Geometry check sheet. Reference: drawing and pictorial views, mm from the part's lowest x, y, z. A direction names the side the tool comes from. Round coordinates to 2 decimals unless told otherwise and drop trailing zeros. Order: outer loops, then holes, each group sorted by start corner. A loop starts at its lowest first (then second) coordinate and runs counter-clockwise, first axis right, second up.
(1) Gauge pin test, flat ends, axial feed: P1, Ø12, axis at x = 15.5, y = 15.5, coming from the +Z side; P2, Ø1.5, axis at x = 29.5, z = 3, coming from the +Y side; P3, Ø4.5, axis at y = 7.5, z = 2.5, coming from the -X side; P4, Ø4, axis at x = 30, y = 5, coming from the -Z side. Record the tip position at first contact, or that the pin passes through.
(2) Cross-section at C-C on z = 5.5. Enter the section's corners in (x, y), and give its area (3 significant figures).
(3) Cross-section at B-B on x = 31.5. Enter the section's corners in (y, z).
(4) Cross-section at D-D on x = 9.5. Enter the section's corners in (y, z), and give its area (3 significant figures).
(5) Draft check along X on the marked faces 4, 5 and 6. Enter one of: pulls with the +X half, pulls with the -X half, needs draft (parallel to the pull), parting line crosses it, or undercut.
(6) Cross-section at A-A on z = 0.5. Enter the section's corners in (x, y).
(7) Thickness scan on L1, parallel to X at y = 9, z = 8; L2, parallel to Y at x = 30, z = 7.5; L3, parallel to X at y = 4, z = 1.75. Record the ranges inside material, lowest first.
(8) Set-up check for the marked faces 1, 2 and 3: record each of +Z, -Z, +X, -X, +Y, -Y from which the full face is reachable in a straight line by a thin tool's end or side.
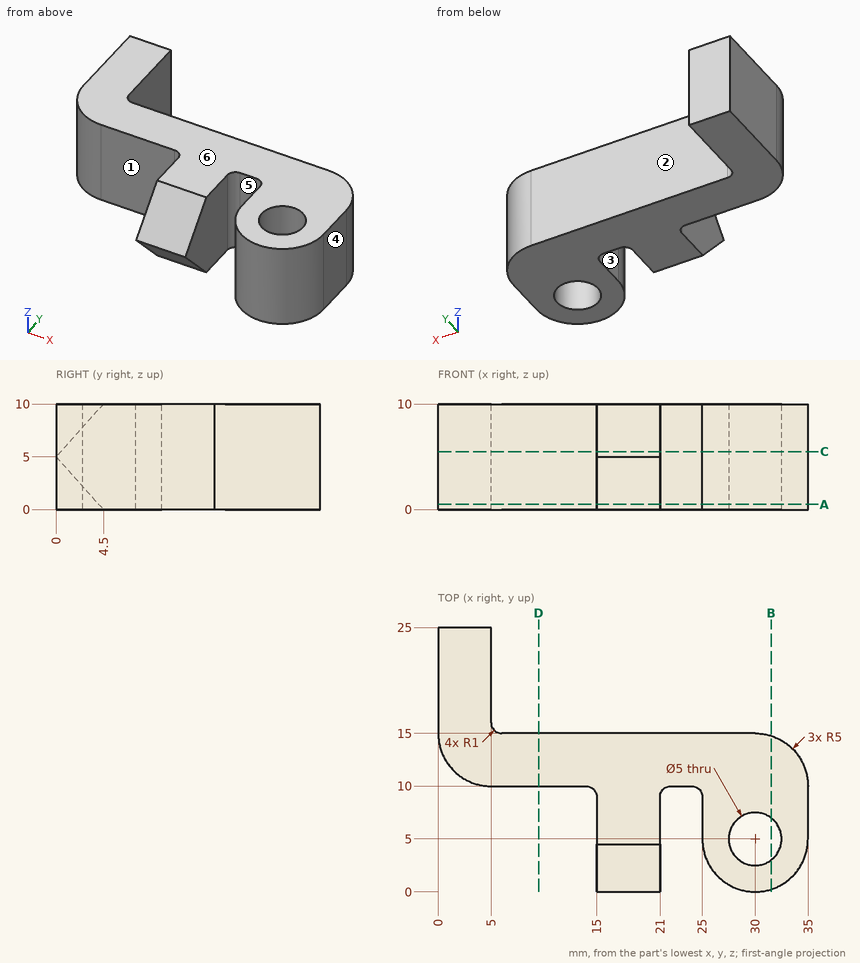
Found:
1. P1: stops at z = 10
1. P2: stops at y = 15
1. P3: stops at x = 14.66
1. P4: passes through
2. outline: (0, 15) arc R5 ccw to (5, 10) - (14, 10) arc R1 cw to (15, 9) - (15, 0.45) - (21, 0.45) - (21, 9) arc R1 cw to (22, 10) - (24, 10) arc R1 cw to (25, 9) - (25, 5) arc R5 ccw to (35, 5) - (35, 10) arc R5 ccw to (30, 15) - (6, 15) arc R1 cw to (5, 16) - (5, 25) - (0, 25) - close; hole circle Ø5 at (30, 5)
2. area: 342 mm2
3. outline: (0.23, 0) - (3, 0) - (3, 10) - (0.23, 10) - close; (7, 0) - (14.77, 0) - (14.77, 10) - (7, 10) - close
4. outline: (10, 0) - (15, 0) - (15, 10) - (10, 10) - close
4. area: 50.0 mm2
5. face 4: pulls with the +X half
5. face 5: undercut
5. face 6: needs draft
6. outline: (0, 15) arc R5 ccw to (5, 10) - (14, 10) arc R1 cw to (15, 9) - (15, 4.05) - (21, 4.05) - (21, 9) arc R1 cw to (22, 10) - (24, 10) arc R1 cw to (25, 9) - (25, 5) arc R5 ccw to (35, 5) - (35, 10) arc R5 ccw to (30, 15) - (6, 15) arc R1 cw to (5, 16) - (5, 25) - (0, 25) - close; hole circle Ø5 at (30, 5)
7. L1: x = 15 to 21, 25 to 35
7. L2: y = 0 to 2.5, 7.5 to 15
7. L3: x = 15 to 21, 25.1 to 27.71, 32.29 to 34.9
8. face 1: +Z, -Z, -X, -Y
8. face 2: +Z, -Z, +X, +Y
8. face 3: +Z, -Z, -Y
